CAD build for the part. Positions are in the model's coordinates, mm. Face numbers are marked on the shaded views. A direction names the side the tool comes from. Give positions to 0.01 mm unless a question says otherwise; leave off trailing zeros. Order: outer loops, then holes, each group sorted by start corner. A loop starts at its lowest first (then second) coordinate and runs counter-clockwise, first axis right, second up.
from build123d import *

# Parameters (mm, degrees)
SKETCH_1_W               = 35
SKETCH_1_H               = 40
EXTRUDE_1_DEPTH          = 9.5
SHELL_1_T                = -1
SKETCH_2_W               = 4
SKETCH_2_H               = 4
EXTRUDE_2_DEPTH          = 8.5
MIRROR_4_COPY_1_SKETCH_W = 4
MIRROR_4_COPY_1_SKETCH_H = 4
MIRROR_4_COPY_1_DEPTH    = 8.5
SKETCH_3_R               = 1.55
CUT_EXTRUDE_1_DEPTH      = 12
MIRROR_6_COPY_1_SKETCH_R = 1.55
MIRROR_6_COPY_1_DEPTH    = 12
SKETCH_6_R               = 1.55
EXTRUDE_3_DEPTH          = 1.5
MIRROR_8_COPY_1_SKETCH_R = 1.55
MIRROR_8_COPY_1_DEPTH    = 1.5
SKETCH_7_W               = 9
SKETCH_7_H               = 1
CUT_EXTRUDE_2_DEPTH      = 3
SKETCH_8_W               = 1
SKETCH_8_H               = 26
CUT_EXTRUDE_3_DEPTH      = 2.2
SKETCH_9_W               = 1
SKETCH_9_H               = 19
CUT_EXTRUDE_4_DEPTH      = 1.2
SKETCH_10_W              = 1
SKETCH_10_H              = 6.5
CUT_EXTRUDE_5_DEPTH      = 2.2
SKETCH_11_W              = 15
SKETCH_11_H              = 1
CUT_EXTRUDE_6_DEPTH      = 2.2
SKETCH_12_W              = 25
SKETCH_12_H              = 4
EXTRUDE_4_DEPTH          = 3.5
SKETCH_13_W              = 21
SKETCH_13_H              = 1.5
CUT_EXTRUDE_7_DEPTH      = 5
CUT_EXTRUDE_8_DEPTH      = 50
SKETCH_15_W              = 15
SKETCH_15_H              = 2
EXTRUDE_5_DEPTH          = 2
FILLET_1_R               = 2
FILLET_2_R               = 1
FILLET_3_R               = 1
FILLET_4_R               = 1
SKETCH_16_W              = 9
SKETCH_16_H              = 1
EXTRUDE_6_DEPTH          = 3


with BuildPart() as part:
    # 草图1 → 凸台-拉伸1 (new body)
    with BuildSketch(Plane.XY):
        Rectangle(SKETCH_1_W, SKETCH_1_H)
    extrude(amount=EXTRUDE_1_DEPTH)

    # 抽壳1
    shell_1_openings = [part.faces().sort_by_distance(p)[0] for p in [
        (0, 0, 9.5),
    ]]
    offset(amount=SHELL_1_T, openings=shell_1_openings, kind=Kind.INTERSECTION)

    # 草图2 → 凸台-拉伸2 (add)
    with BuildSketch(Plane.XY.offset(1)):
        with Locations((-14.5, 17)):
            Rectangle(SKETCH_2_W, SKETCH_2_H)
    extrude_2 = extrude(amount=EXTRUDE_2_DEPTH)

    # 镜向3: 凸台-拉伸2 across plane
    add(extrude_2.mirror(Plane.ZX))

    # 镜向4: 凸台-拉伸2 across plane
    add(extrude_2.mirror(Plane(origin=(0, 0, 0), x_dir=(0, 0, 1), z_dir=(1, 0, 0))))

    # 镜向4 copy 1 sketch → 镜向4 copy 1 (add)
    with BuildSketch(Plane(origin=(0, 0, 1), x_dir=(-1, 0, 0), z_dir=(0, 0, 1))):
        with Locations((-14.5, 17)):
            Rectangle(MIRROR_4_COPY_1_SKETCH_W, MIRROR_4_COPY_1_SKETCH_H)
    extrude(amount=MIRROR_4_COPY_1_DEPTH)

    # 草图3 → 切除-拉伸1 (cut)
    with BuildSketch(Plane(origin=(0, 0, 0), x_dir=(-1, 0, 0), z_dir=(0, 0, -1))):
        with Locations((-14.7, 17.2)):
            Circle(SKETCH_3_R)
    cut_extrude_1 = extrude(amount=-CUT_EXTRUDE_1_DEPTH, mode=Mode.SUBTRACT)

    # 镜向5: 切除-拉伸1 across plane
    add(cut_extrude_1.mirror(Plane.ZX), mode=Mode.SUBTRACT)

    # 镜向6: 切除-拉伸1 across plane
    add(cut_extrude_1.mirror(Plane(origin=(0, 0, 0), x_dir=(0, 0, 1), z_dir=(1, 0, 0))), mode=Mode.SUBTRACT)

    # 镜向6 copy 1 sketch → 镜向6 copy 1 (cut)
    with BuildSketch(Plane(origin=(0, 0, 0), x_dir=(1, 0, 0), z_dir=(0, 0, -1))):
        with Locations((-14.7, 17.2)):
            Circle(MIRROR_6_COPY_1_SKETCH_R)
    extrude(amount=-MIRROR_6_COPY_1_DEPTH, mode=Mode.SUBTRACT)

    # 草图6 → 凸台-拉伸3 (add)
    with BuildSketch(Plane(origin=(0, 0, 0), x_dir=(-1, 0, 0), z_dir=(0, 0, -1))):
        with Locations((-14.7, 17.2)):
            Circle(SKETCH_6_R)
    extrude_3 = extrude(amount=-EXTRUDE_3_DEPTH)

    # 镜向7: 凸台-拉伸3 across plane
    add(extrude_3.mirror(Plane.ZX))

    # 镜向8: 凸台-拉伸3 across plane
    add(extrude_3.mirror(Plane(origin=(0, 0, 0), x_dir=(0, 0, 1), z_dir=(1, 0, 0))))

    # 镜向8 copy 1 sketch → 镜向8 copy 1 (add)
    with BuildSketch(Plane(origin=(0, 0, 0), x_dir=(1, 0, 0), z_dir=(0, 0, -1))):
        with Locations((-14.7, 17.2)):
            Circle(MIRROR_8_COPY_1_SKETCH_R)
    extrude(amount=-MIRROR_8_COPY_1_DEPTH)

    # 草图7 → 切除-拉伸2 (cut)
    with BuildSketch(Plane.XY.offset(9.5)):
        with Locations((-5, 19.5)):
            Rectangle(SKETCH_7_W, SKETCH_7_H)
    cut_extrude_2 = extrude(amount=-CUT_EXTRUDE_2_DEPTH, mode=Mode.SUBTRACT)

    # 草图8 → 切除-拉伸3 (cut)
    with BuildSketch(Plane.XY.offset(9.5)):
        with Locations((-17, 0)):
            Rectangle(SKETCH_8_W, SKETCH_8_H)
    extrude(amount=-CUT_EXTRUDE_3_DEPTH, mode=Mode.SUBTRACT)

    # 草图9 → 切除-拉伸4 (cut)
    with BuildSketch(Plane.XY.offset(9.5)):
        with Locations((17, -4.5)):
            Rectangle(SKETCH_9_W, SKETCH_9_H)
    extrude(amount=-CUT_EXTRUDE_4_DEPTH, mode=Mode.SUBTRACT)

    # 草图10 → 切除-拉伸5 (cut)
    with BuildSketch(Plane.XY.offset(9.5)):
        with Locations((17, 9.55)):
            Rectangle(SKETCH_10_W, SKETCH_10_H)
    extrude(amount=-CUT_EXTRUDE_5_DEPTH, mode=Mode.SUBTRACT)

    # 草图11 → 切除-拉伸6 (cut)
    with BuildSketch(Plane.XY.offset(9.5)):
        with Locations((0, -19.5)):
            Rectangle(SKETCH_11_W, SKETCH_11_H)
    extrude(amount=-CUT_EXTRUDE_6_DEPTH, mode=Mode.SUBTRACT)

    # 草图12 → 凸台-拉伸4 (add)
    with BuildSketch(Plane.XZ.offset(20)):
        with Locations((0, 2)):
            Rectangle(SKETCH_12_W, SKETCH_12_H)
    extrude_4 = extrude(amount=EXTRUDE_4_DEPTH)

    # 草图13 → 切除-拉伸7 (cut)
    with BuildSketch(Plane.XY.offset(4)):
        with Locations((0, -20.75)):
            Rectangle(SKETCH_13_W, SKETCH_13_H)
    cut_extrude_7 = extrude(amount=-CUT_EXTRUDE_7_DEPTH, mode=Mode.SUBTRACT)

    # 草图14 → 切除-拉伸8 (cut)
    with BuildSketch(Plane(origin=(12.5, 0, 0), x_dir=(0, 0, -1), z_dir=(1, 0, 0))):
        Polygon((-2, -23.5), (-4, -23.5), (-4, -21.75), (-4, -20), align=None)
    cut_extrude_8 = extrude(amount=-CUT_EXTRUDE_8_DEPTH, mode=Mode.SUBTRACT)

    # 镜向11: 凸台-拉伸4, 切除-拉伸7, 切除-拉伸8 across plane
    add(extrude_4.mirror(Plane.ZX))
    add(cut_extrude_7.mirror(Plane.ZX), mode=Mode.SUBTRACT)
    add(cut_extrude_8.mirror(Plane.ZX), mode=Mode.SUBTRACT)

    # 草图15 → 凸台-拉伸5 (add)
    with BuildSketch(Plane.XZ.offset(20)):
        with Locations((0, 6.3)):
            Rectangle(SKETCH_15_W, SKETCH_15_H)
    extrude(amount=EXTRUDE_5_DEPTH)

    # 圆角1
    fillet_1_edges = [part.edges().sort_by_distance(p)[0] for p in [
        (-17.5, 20, 4.75),
        (17.5, 20, 4.75),
        (17.5, -20, 4.75),
        (-17.5, -20, 4.75),
    ]]
    fillet(fillet_1_edges, radius=FILLET_1_R)

    # 圆角2
    fillet_2_edges = [part.edges().sort_by_distance(p)[0] for p in [
        (14, -20, 0),
        (0, -20, 0),
        (-14, 20, 0),
        (0, 20, 0),
        (-17.5, 0, 0),
        (14, 20, 0),
        (17.5, 0, 0),
        (-14, -20, 0),
        (-16.914213562, -19.414213562, 0),
        (16.914213562, -19.414213562, 0),
        (16.914213562, 19.414213562, 0),
        (-16.914213562, 19.414213562, 0),
    ]]
    fillet(fillet_2_edges, radius=FILLET_2_R)

    # 圆角3
    fillet_3_edges = [part.edges().sort_by_distance(p)[0] for p in [
        (12.5, -23.5, 1),
        (-12.5, -23.5, 1),
        (12.5, 23.5, 1),
        (-12.5, 23.5, 1),
    ]]
    fillet(fillet_3_edges, radius=FILLET_3_R)

    # 圆角4
    fillet_4_edges = [part.edges().sort_by_distance(p)[0] for p in [
        (-7.5, -22, 6.3),
        (0, -22, 5.3),
        (7.5, -22, 6.3),
    ]]
    fillet(fillet_4_edges, radius=FILLET_4_R)

    # 镜向12: 切除-拉伸2 across plane
    add(cut_extrude_2.mirror(Plane(origin=(0, 0, 0), x_dir=(0, 0, 1), z_dir=(1, 0, 0))), mode=Mode.SUBTRACT)

    # 草图16 → 凸台-拉伸6 (add)
    with BuildSketch(Plane.XY.offset(6.5)):
        with Locations((-5, 19.5)):
            Rectangle(SKETCH_16_W, SKETCH_16_H)
    extrude(amount=EXTRUDE_6_DEPTH)


solid = part.part
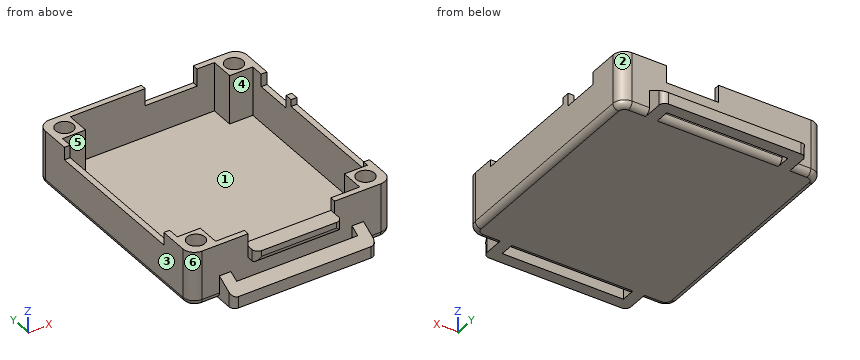
1. Mould opens along Y. For the marked faces 3, 4, 5 and 6 say: released by +Y, released by -Y, zero draft, split by the parting line, or undercut.
2. Saw through at A-A on x = 1. Give the cut face in (y, z), plus the area to 3 significant figures.
3. Saw through at D-D on y = 11. Give the cut face in (x, z), plus the area to 3 significant figures.
4. Pin check, flat tips, straight feed: P1, Ø1.2, axis at y = 21, z = 2.5, coming from the -X side; P2, Ø4, axis at y = -20.5, z = 2, coming from the +X side; P3, Ø0.8, axis at y = 19.5, z = 8.5, coming from the -X side. Stop position of each tip, or through.
5. Saw through at C-C on x = -14.7. Give the cut face in (y, z).
6. Wall check: line 1 (X direction, y = -17.2, z = 5.25); line 2 (Y direction, x = 1, z = 1.25); line 3 (Y direction, x = 14.7, z = 6.5). Give the ranges that are in metal, low to high.
7. 3-axis set-ups, long thin cutter, end or side, ignore diameter. For the marked faces 1 and 2: which of +Z, -Z, +X, -X, +Y, -Y reach the whole face in a straight line?
8. Saw through at B-B on y = -17.2. Give the cut face in (x, z), plus the area to 3 significant figures.
Reported:
1. face 3: zero draft
1. face 4: undercut
1. face 5: undercut
1. face 6: released by -Y
2. outline: (-23.5, 0) - (-21.5, 0) - (-21.5, 3.14) - (-23.5, 2) - close; (-22, 6.3) arc R1 ccw to (-21, 5.3) - (-20, 5.3) - (-20, 1) arc R1 ccw to (-19, 0) - (19, 0) arc R1 ccw to (20, 1) - (20, 6.5) - (19, 6.5) - (19, 1) - (-19, 1) - (-19, 7.3) - (-22, 7.3) - close; (21.5, 0) - (23.5, 0) - (23.5, 2) - (21.5, 3.14) - close
2. area: 65.4 mm2
3. outline: (-17.5, 1) arc R1 ccw to (-16.5, 0) - (16.5, 0) arc R1 ccw to (17.5, 1) - (17.5, 7.3) - (16.5, 7.3) - (16.5, 1) - (-16.5, 1) - (-16.5, 7.3) - (-17.5, 7.3) - close
3. area: 47.2 mm2
4. P1: stops at x = -12.5
4. P2: stops at x = 17.44
4. P3: stops at x = -17.17
5. outline: (-20, 1) arc R1 ccw to (-19, 0) - (19, 0) arc R1 ccw to (20, 1) - (20, 9.5) - (18.75, 9.5) - (18.75, 1.5) - (15.65, 1.5) - (15.65, 9.5) - (15, 9.5) - (15, 1) - (-15, 1) - (-15, 9.5) - (-15.65, 9.5) - (-15.65, 1.5) - (-18.75, 1.5) - (-18.75, 9.5) - (-20, 9.5) - close
6. line 1: x = -17.5 to -16.25, -13.15 to -12.5, 12.5 to 13.15, 16.25 to 17.5
6. line 2: y = -23.5 to -21.5, -20 to -19, 19 to 20, 21.5 to 23.5
6. line 3: y = -20 to -18.75, -15.65 to -15, 15 to 15.65, 18.75 to 20
7. face 1: +Z
7. face 2: +Z, -Z, +X, +Y
8. outline: (-17.5, 1) arc R1 ccw to (-16.5, 0) - (16.5, 0) arc R1 ccw to (17.5, 1) - (17.5, 9.5) - (16.25, 9.5) - (16.25, 1.5) - (13.15, 1.5) - (13.15, 9.5) - (12.5, 9.5) - (12.5, 1) - (-12.5, 1) - (-12.5, 9.5) - (-13.15, 9.5) - (-13.15, 1.5) - (-16.25, 1.5) - (-16.25, 9.5) - (-17.5, 9.5) - close
8. area: 70.0 mm2
